```python
from build123d import *

# Parameters (mm, degrees)
SKETCH1_R           = 10
BOSS_EXTRUDE2_DEPTH = 109
SKETCH3_W           = 10
SKETCH3_H           = 5
CUT_EXTRUDE1_DEPTH  = 20


with BuildPart() as part:
    # Sketch1 → Boss-Extrude2 (new body)
    with BuildSketch(Plane(origin=(0, 0, 0), x_dir=(1, 0, 0), z_dir=(0, 1, 0))):
        Circle(SKETCH1_R)
    extrude(amount=BOSS_EXTRUDE2_DEPTH)

    # Sketch3 → Cut-Extrude1 (cut)
    with BuildSketch(Plane.XZ):
        with Locations((10, 0)):
            Rectangle(SKETCH3_W, SKETCH3_H)
    extrude(amount=-CUT_EXTRUDE1_DEPTH, mode=Mode.SUBTRACT)


solid = part.part
```
Geometry check sheet. Reference: the model listing, model coordinates, mm. A direction names the side the tool comes from. Give positions to 0.01 mm unless a question says otherwise; leave off trailing zeros. Loops run counter-clockwise (first coordinate to the right, second up) from the corner with the lowest first, then second, coordinate; pieces in that order, holes last. Notation, with made-up numbers: M 26,60 L 82,60 A12 ccw 82,77 Z; hole C 19.25,77.25 d6. An arc over 180 degrees is marked long. Write item = value, one per line. Start each with the question number.
1. Section check A-A, the plane z = 6. Enter the section's corners in (x, y).
2. Draft check along Z on faces 1 (the face through (0, 109, 0)), 2 (the face through (-2.17, 53.74, 9.76)), 3 (the face through (7, 20, 0)). Enter one of: +Z half, -Z half, draft (parallel to the pull), parting line (faces both ways), or undercut.
3. Thickness scan on probe 1 along Z at (x, y) = (-0.25, 49); probe 2 along Z at (x, y) = (6.5, 10); probe 3 along X at (y, z) = (62.5, -7). Record the ranges inside material, lowest first.
4. Section check C-C, the plane x = 7.25. Enter the section's corners in (y, z), plus the area to 3 significant figures.
5. Tool access check on faces 4 (the face through (5, 10, 0)), 5 (the face through (0, 0, 0)). Record the directions out of +Z, -Z, +X, -X, +Y, -Y that give a thin tool (end or side, any length) a straight path to the whole face; none if there is none.
6. Section check D-D, the plane z = 0. Enter the section's corners in (x, y).
7. Go/stop test with flat-tipped pins: P1, Ø6, axis at x = -6.5, y = 45.5, coming from the -Z side; P2, Ø5, axis at x = -4.5, y = 62, coming from the +Z side; P3, Ø2.5, axis at x = 6.5, y = 12.5, coming from the -Z side. Record where each tip stops, or that it passes through.
8. Section check B-B, the plane y = 89. Enter the section's corners in (x, z).
Values follow:
q1.outline = M -8,0 L 8,0 L 8,109 L -8,109 Z
q2.face_1 = draft
q2.face_2 = parting line
q2.face_3 = undercut
q3.probe_1 = -10 to 10
q3.probe_2 = -7.6 to -2.5, 2.5 to 7.6
q3.probe_3 = -7.14 to 7.14
q4.outline = M 0,-6.89 L 109,-6.89 L 109,6.89 L 0,6.89 L 0,2.5 L 20,2.5 L 20,-2.5 L 0,-2.5 Z
q4.area = 1,400 mm^2
q5.face_4 = +X, -Y
q5.face_5 = +Z, -Z, +X, -X, -Y
q6.outline = M -10,0 L 5,0 L 5,20 L 10,20 L 10,109 L -10,109 Z
q7.P1 = -9.37
q7.P2 = 9.8
q7.P3 = -8.51
q8.outline = C 0,0 d20
